from build123d import *

# Parameters (mm, degrees)
F1_DEPTH = 25


with BuildPart() as f1:
    # F0 (on Top) → F1 (new body)
    with BuildSketch(Plane.XY):
        with BuildLine():
            ThreePointArc((-13.25, -22.9496732003), (13.25, -22.9496732003), (26.5, 0))
            ThreePointArc((26.5, 0), (22.9496732003, 13.25), (13.25, 22.9496732003))
            ThreePointArc((13.25, 22.9496732003), (9.6996732003, 9.6996732003), (0, 0))
            ThreePointArc((0, 0), (-3.5503267997, -13.25), (-13.25, -22.9496732003))
        make_face()
        with BuildLine():
            ThreePointArc((0, 0), (9.6996732003, 9.6996732003), (13.25, 22.9496732003))
            ThreePointArc((13.25, 22.9496732003), (0, 26.5), (-13.25, 22.9496732003))
            ThreePointArc((-13.25, 22.9496732003), (-3.5503267997, 13.25), (0, 0))
        make_face()
        with BuildLine():
            ThreePointArc((-13.25, 22.9496732003), (0, 26.5), (13.25, 22.9496732003))
            ThreePointArc((13.25, 22.9496732003), (-13.25, 49.4496732003), (-39.75, 22.9496732003))
            ThreePointArc((-39.75, 22.9496732003), (-26.5, 26.5), (-13.25, 22.9496732003))
        make_face()
        with BuildLine():
            ThreePointArc((-39.75, 22.9496732003), (-49.4496732003, -13.25), (-13.25, -22.9496732003))
            ThreePointArc((-13.25, -22.9496732003), (-22.9496732003, -13.25), (-26.5, 0))
            ThreePointArc((-26.5, 0), (-36.1996732003, 9.6996732003), (-39.75, 22.9496732003))
        make_face()
        with BuildLine():
            ThreePointArc((-26.5, 0), (-22.9496732003, -13.25), (-13.25, -22.9496732003))
            ThreePointArc((-13.25, -22.9496732003), (-3.5503267997, -13.25), (0, 0))
            ThreePointArc((0, 0), (-13.25, -3.5503267997), (-26.5, 0))
        make_face()
        with BuildLine():
            ThreePointArc((-26.5, 0), (-22.9496732003, 13.25), (-13.25, 22.9496732003))
            ThreePointArc((-13.25, 22.9496732003), (-26.5, 26.5), (-39.75, 22.9496732003))
            ThreePointArc((-39.75, 22.9496732003), (-36.1996732003, 9.6996732003), (-26.5, 0))
        make_face()
    extrude(amount=F1_DEPTH)


solid = f1.part
Geometry: final body of the model. Coordinates: model frame, mm. A direction names the side the tool comes from. Give positions to 0.01 mm unless a question says otherwise; leave off trailing zeros. Loops run counter-clockwise (first coordinate to the right, second up) from the corner with the lowest first, then second, coordinate; pieces in that order, holes last. Notation, with made-up numbers: (-31, 43.25) - (-11, 43.25) arc R16 cw to (-11, 53.25) - close; hole circle Ø5 at (-5, 60). An arc over 180 degrees is marked (long way). Answer as CSV lines item,"result". Start each with the question number.
1. Draft query along X for faces 3 (the face through (-12.667, 49.443, 12.325)), 4 (the face through (-14, -5, 25)), 5 (the face through (-3.65, 13.42, 12.32)). Return one class per face: released by +X, released by -X, zero draft, split by the parting line, or undercut.
2. Pin query (flat end, axial travel): P1, Ø6, axis at y = -13.5, z = 7, coming from the -X side; P2, Ø12, axis at x = -9.5, z = 16, coming from the -Y side; P3, Ø12, axis at x = 16.5, z = 4.5, coming from the +Y side (3 decimals). Return the tip coordinate at first contact, or that it passes through.
3. Reachability of faces 1 (the face through (-13.06, -3.55, 12.32)), 2 (the face through (-14, -5, 0)) from +Z, -Z, +X, -X, +Y, -Y: full face, straight path, thin tool, end or side. Return the list, or none.
4. Section C-C, the plane y = 11.5. Return loops of the section in (x, z), plus the area to 4 significant figures.
5. Section D-D, the plane y = 44. Return loops of the section in (x, z).
6. Section B-B, the plane z = 12.5. Return loops of the section in (x, y).
7. Section A-A, the plane x = -1. Return loops of the section in (y, z), plus the area to 3 significant figures.
8. Ray query, L1, parallel to X at y = 0.5, z = 18.5; L2, parallel to Y at x = -13, z = 22.5; L3, parallel to X at y = 6, z = 8.5. Return the intervals inside material, ascending.
Answers:
1,face 3,"split by the parting line"
1,face 4,"zero draft"
1,face 5,"undercut"
2,P1,"stops at x = -50.83"
2,P2,"stops at y = -26.27"
2,P3,"stops at y = 34.705"
3,face 1,"+Z, -Z"
3,face 2,"-Z, +X, -X, +Y, -Y"
4,outline,"(-50.37, 0) - (-23.87, 0) - (-23.87, 25) - (-50.37, 25) - close; (-2.63, 0) - (23.87, 0) - (23.87, 25) - (-2.63, 25) - close"
4,area,"1,325 mm2"
5,outline,"(-29.35, 0) - (2.85, 0) - (2.85, 25) - (-29.35, 25) - close"
6,outline,"(-39.75, 22.95) arc R26.5 ccw to (-13.25, -22.95) arc R26.5 ccw to (13.25, 22.95) arc R26.5 ccw to start; hole (-26.5, 0) arc R26.5 ccw to (0, 0) arc R26.5 ccw to (-13.25, 22.95) arc R26.5 ccw to start"
7,outline,"(-26.48, 0) - (-0.55, 0) - (-0.55, 25) - (-26.48, 25) - close; (7.21, 0) - (46.45, 0) - (46.45, 25) - (7.21, 25) - close"
7,area,"1,630 mm2"
8,L1,"x = -53 to -26.5, 0 to 26.5"
8,L2,"y = -23.09 to -3.55, 22.8 to 49.45"
8,L3,"x = -52.31 to -25.81, -0.69 to 25.81"
